Here's how the part is built. I have some questions about the finished solid (model axes, mm). Face numbers are marked on the shaded views. A direction names the side the tool comes from. Round coordinates to 2 decimals unless told otherwise and drop trailing zeros. Write each loop counter-clockwise with the first axis right and the second up, starting at its lowest first coordinate (ties: lowest second). Pieces come first, ordered by that corner, then holes. Notation, with made-up numbers: (41, 65.25) - (54, 65.25) arc R11 ccw to (54, 80.25) - close; hole circle Ø11 at (-15, -1.5). An arc over 180 degrees is marked (long way). One line per item, written item: value. Start each with the question number.
Item 1: Imagine slicing it at D-D, the plane z = 44. Count the separate pieces of the cut face and the enclosed holes in it, then the cut area to 3 significant figures.
Item 2: For the marked faces 1 and 2, which set-ups out of +Z, -Z, +X, -X, +Y, -Y let a thin tool reach every point of the face, with its end or its side?
Item 3: Thinking about a two-plate mould opening in X: for the marked faces 3, 4 and 5, which applies, released by +X, released by -X, zero draft, split by the parting line, or undercut?
Item 4: Imagine slicing it at A-A, the plane y = 0. Please give me the cut outline in (x, z).
Item 5: Imagine slicing it at C-C, the plane x = -42. Please give me the cut outline in (y, z).
Item 6: If I drill on line 1 (X direction, y = 40, z = 47.5); line 2 (X direction, y = 0.5, z = 47.75); line 3 (X direction, y = -34.5, z = 48.5), over which ranges is the centre line in solid material (lowest first)?
Item 7: For P1, Ø5, axis at x = -17.5, z = 49.5, coming from the +Y side; P2, Ø2, axis at y = -38.5, z = 46.5, coming from the +X side; P3, Ø2, axis at x = 43.5, z = 46, coming from the -Y side, each with a flat end and sliding along its axis, tell me the tip position at first contact or that it passes through.
```python
from build123d import *

# Parameters (mm, degrees)
CYLINDER469_R               = 1.5
CYLINDER469_DEPTH           = 100
CYLINDER472_R               = 1.5
CYLINDER472_DEPTH           = 100
CYLINDER472_ROLL_ANGLE      = -0.500355
CYLINDER472_PITCH_ANGLE     = 0.967193
CYLINDER472_PLACEMENT_ANGLE = 144.93646
CYLINDER481_R               = 1.5
CYLINDER481_DEPTH           = 100
CYLINDER476_R               = 1.5
CYLINDER476_DEPTH           = 100
CYLINDER476_PLACEMENT_ANGLE = 225
CYLINDER470_R               = 1.5
CYLINDER470_DEPTH           = 100
CYLINDER475_R               = 1.5
CYLINDER475_DEPTH           = 100
CYLINDER475_PLACEMENT_ANGLE = 45
CYLINDER479_R               = 1.5
CYLINDER479_DEPTH           = 100
CYLINDER479_ROLL_ANGLE      = 0.146073
CYLINDER479_PITCH_ANGLE     = 1.079101
CYLINDER479_PLACEMENT_ANGLE = -9.939308
CYLINDER471_R               = 1.5
CYLINDER471_DEPTH           = 100
CYLINDER471_PLACEMENT_ANGLE = 45
CYLINDER468_R               = 8
CYLINDER468_DEPTH           = 18
CYLINDER480_R               = 8
CYLINDER480_DEPTH           = 18
CYLINDER480_PLACEMENT_ANGLE = 225
CYLINDER483_R               = 8
CYLINDER483_DEPTH           = 18
CYLINDER482_R               = 8
CYLINDER482_DEPTH           = 18
CYLINDER482_ROLL_ANGLE      = -0.500355
CYLINDER482_PITCH_ANGLE     = 0.967193
CYLINDER482_PLACEMENT_ANGLE = 144.93646
CYLINDER474_R               = 8
CYLINDER474_DEPTH           = 18
CYLINDER478_R               = 8
CYLINDER478_DEPTH           = 18
CYLINDER478_PLACEMENT_ANGLE = 45
CYLINDER473_R               = 8
CYLINDER473_DEPTH           = 18
CYLINDER473_ROLL_ANGLE      = 0.146073
CYLINDER473_PITCH_ANGLE     = 1.079101
CYLINDER473_PLACEMENT_ANGLE = -9.939308
CYLINDER477_R               = 8
CYLINDER477_DEPTH           = 18
CYLINDER477_PLACEMENT_ANGLE = 45
TUBE025_R                   = 58
TUBE025_R_2                 = 30
TUBE025_DEPTH               = 10


with BuildPart() as obj1:
    # Cylinder469 → Cylinder469 (new body)
    with BuildSketch(Plane(origin=(38.80294, -16.072704, 0), x_dir=(0, 1, 0), z_dir=(0, 0, 1))):
        Circle(CYLINDER469_R)
    extrude(amount=CYLINDER469_DEPTH)


with BuildPart() as obj2:
    # Cylinder472 → Cylinder472 (new body)
    with BuildSketch(Plane.XY):
        Circle(CYLINDER472_R)
    extrude(amount=CYLINDER472_DEPTH)


with BuildPart() as obj2_1:
    # Cylinder472 roll: moved
    add(obj2.part.rotate(Axis((0, 0, 0), (1, 0, 0)), CYLINDER472_ROLL_ANGLE))


with BuildPart() as obj2_2:
    # Cylinder472 pitch: moved
    add(obj2_1.part.rotate(Axis((0, 0, 0), (0, 1, 0)), CYLINDER472_PITCH_ANGLE))


with BuildPart() as obj2_3:
    # Cylinder472 placement: moved
    add(obj2_2.part.moved(Location((35.440039, 22.530677, 0.610113))).rotate(Axis((35.440039, 22.530677, 0.610113), (0, 0, 1)), CYLINDER472_PLACEMENT_ANGLE))


with BuildPart() as obj3:
    # Cylinder481 → Cylinder481 (new body)
    with BuildSketch(Plane(origin=(16.072704, 38.80294, 0), x_dir=(-1, 0, 0), z_dir=(0, 0, 1))):
        Circle(CYLINDER481_R)
    extrude(amount=CYLINDER481_DEPTH)


with BuildPart() as obj4:
    # Cylinder476 → Cylinder476 (new body)
    with BuildSketch(Plane.XY):
        Circle(CYLINDER476_R)
    extrude(amount=CYLINDER476_DEPTH)


with BuildPart() as obj4_1:
    # Cylinder476 placement: moved
    add(obj4.part.moved(Location((-16.072704, 38.80294, 0))).rotate(Axis((-16.072704, 38.80294, 0), (0, 0, 1)), CYLINDER476_PLACEMENT_ANGLE))


with BuildPart() as obj5:
    # Cylinder470 → Cylinder470 (new body)
    with BuildSketch(Plane(origin=(-38.80294, 16.072704, 0), x_dir=(0, -1, 0), z_dir=(0, 0, 1))):
        Circle(CYLINDER470_R)
    extrude(amount=CYLINDER470_DEPTH)


with BuildPart() as obj6:
    # Cylinder475 → Cylinder475 (new body)
    with BuildSketch(Plane.XY):
        Circle(CYLINDER475_R)
    extrude(amount=CYLINDER475_DEPTH)


with BuildPart() as obj6_1:
    # Cylinder475 placement: moved
    add(obj6.part.moved(Location((-38.80294, -16.072704, 0))).rotate(Axis((-38.80294, -16.072704, 0), (0, 0, -1)), CYLINDER475_PLACEMENT_ANGLE))


with BuildPart() as obj7:
    # Cylinder479 → Cylinder479 (new body)
    with BuildSketch(Plane.XY):
        Circle(CYLINDER479_R)
    extrude(amount=CYLINDER479_DEPTH)


with BuildPart() as obj7_1:
    # Cylinder479 roll: moved
    add(obj7.part.rotate(Axis((0, 0, 0), (1, 0, 0)), CYLINDER479_ROLL_ANGLE))


with BuildPart() as obj7_2:
    # Cylinder479 pitch: moved
    add(obj7_1.part.rotate(Axis((0, 0, 0), (0, 1, 0)), CYLINDER479_PITCH_ANGLE))


with BuildPart() as obj7_3:
    # Cylinder479 placement: moved
    add(obj7_2.part.moved(Location((-22.528054, -35.446371, 0.203785))).rotate(Axis((-22.528054, -35.446371, 0.203785), (0, 0, 1)), CYLINDER479_PLACEMENT_ANGLE))


with BuildPart() as compound338:
    # Cylinder471 → Cylinder471 (new body)
    with BuildSketch(Plane.XY):
        Circle(CYLINDER471_R)
    extrude(amount=CYLINDER471_DEPTH)


with BuildPart() as compound338_1:
    # Cylinder471 placement: moved
    add(compound338.part.moved(Location((16.072704, -38.80294, 0))).rotate(Axis((16.072704, -38.80294, 0), (0, 0, 1)), CYLINDER471_PLACEMENT_ANGLE))

    # Compound338: union obj1, obj2, obj3, obj4, obj5, obj6, obj7
    add(obj1.part)
    add(obj2_3.part)
    add(obj3.part)
    add(obj4_1.part)
    add(obj5.part)
    add(obj6_1.part)
    add(obj7_3.part)


with BuildPart() as obj8:
    # Cylinder468 → Cylinder468 (new body)
    with BuildSketch(Plane(origin=(-38.798949, 16.072537, 43), x_dir=(0, -1, 0), z_dir=(0, 0, 1))):
        Circle(CYLINDER468_R)
    extrude(amount=CYLINDER468_DEPTH)


with BuildPart() as obj9:
    # Cylinder480 → Cylinder480 (new body)
    with BuildSketch(Plane.XY):
        Circle(CYLINDER480_R)
    extrude(amount=CYLINDER480_DEPTH)


with BuildPart() as obj9_1:
    # Cylinder480 placement: moved
    add(obj9.part.moved(Location((-16.07, 38.8, 43))).rotate(Axis((-16.07, 38.8, 43), (0, 0, 1)), CYLINDER480_PLACEMENT_ANGLE))


with BuildPart() as obj10:
    # Cylinder483 → Cylinder483 (new body)
    with BuildSketch(Plane(origin=(16.072537, 38.798949, 43), x_dir=(-1, 0, 0), z_dir=(0, 0, 1))):
        Circle(CYLINDER483_R)
    extrude(amount=CYLINDER483_DEPTH)


with BuildPart() as obj11:
    # Cylinder482 → Cylinder482 (new body)
    with BuildSketch(Plane.XY):
        Circle(CYLINDER482_R)
    extrude(amount=CYLINDER482_DEPTH)


with BuildPart() as obj11_1:
    # Cylinder482 roll: moved
    add(obj11.part.rotate(Axis((0, 0, 0), (1, 0, 0)), CYLINDER482_ROLL_ANGLE))


with BuildPart() as obj11_2:
    # Cylinder482 pitch: moved
    add(obj11_1.part.rotate(Axis((0, 0, 0), (0, 1, 0)), CYLINDER482_PITCH_ANGLE))


with BuildPart() as obj11_3:
    # Cylinder482 placement: moved
    add(obj11_2.part.moved(Location((34.627801, 22.637113, 43.602309))).rotate(Axis((34.627801, 22.637113, 43.602309), (0, 0, 1)), CYLINDER482_PLACEMENT_ANGLE))


with BuildPart() as obj12:
    # Cylinder474 → Cylinder474 (new body)
    with BuildSketch(Plane(origin=(38.798949, -16.072537, 43), x_dir=(0, 1, 0), z_dir=(0, 0, 1))):
        Circle(CYLINDER474_R)
    extrude(amount=CYLINDER474_DEPTH)


with BuildPart() as obj13:
    # Cylinder478 → Cylinder478 (new body)
    with BuildSketch(Plane.XY):
        Circle(CYLINDER478_R)
    extrude(amount=CYLINDER478_DEPTH)


with BuildPart() as obj13_1:
    # Cylinder478 placement: moved
    add(obj13.part.moved(Location((16.07, -38.8, 43))).rotate(Axis((16.07, -38.8, 43), (0, 0, 1)), CYLINDER478_PLACEMENT_ANGLE))


with BuildPart() as obj14:
    # Cylinder473 → Cylinder473 (new body)
    with BuildSketch(Plane.XY):
        Circle(CYLINDER473_R)
    extrude(amount=CYLINDER473_DEPTH)


with BuildPart() as obj14_1:
    # Cylinder473 roll: moved
    add(obj14.part.rotate(Axis((0, 0, 0), (1, 0, 0)), CYLINDER473_ROLL_ANGLE))


with BuildPart() as obj14_2:
    # Cylinder473 pitch: moved
    add(obj14_1.part.rotate(Axis((0, 0, 0), (0, 1, 0)), CYLINDER473_PITCH_ANGLE))


with BuildPart() as obj14_3:
    # Cylinder473 placement: moved
    add(obj14_2.part.moved(Location((-21.748471, -35.690226, 43.196026))).rotate(Axis((-21.748471, -35.690226, 43.196026), (0, 0, 1)), CYLINDER473_PLACEMENT_ANGLE))


with BuildPart() as compound336:
    # Cylinder477 → Cylinder477 (new body)
    with BuildSketch(Plane.XY):
        Circle(CYLINDER477_R)
    extrude(amount=CYLINDER477_DEPTH)


with BuildPart() as compound336_1:
    # Cylinder477 placement: moved
    add(compound336.part.moved(Location((-38.8, -16.07, 43))).rotate(Axis((-38.8, -16.07, 43), (0, 0, -1)), CYLINDER477_PLACEMENT_ANGLE))

    # Compound336: union obj8, obj9, obj10, obj11, obj12, obj13, obj14
    add(obj8.part)
    add(obj9_1.part)
    add(obj10.part)
    add(obj11_3.part)
    add(obj12.part)
    add(obj13_1.part)
    add(obj14_3.part)


with BuildPart() as compound336_2:
    # Compound336 placement: moved
    add(compound336_1.part.moved(Location((0, 0, 3))))


with BuildPart() as obj15:
    # Tube025 → Tube025 (new body)
    with BuildSketch(Plane.XY.offset(42)):
        Circle(TUBE025_R)
        Circle(TUBE025_R_2, mode=Mode.SUBTRACT)
    extrude(amount=TUBE025_DEPTH)

    # Cut173: cut Compound336
    add(compound336_2.part, mode=Mode.SUBTRACT)

    # Cut174: cut Compound338
    add(compound338_1.part, mode=Mode.SUBTRACT)


solid = obj15.part
```
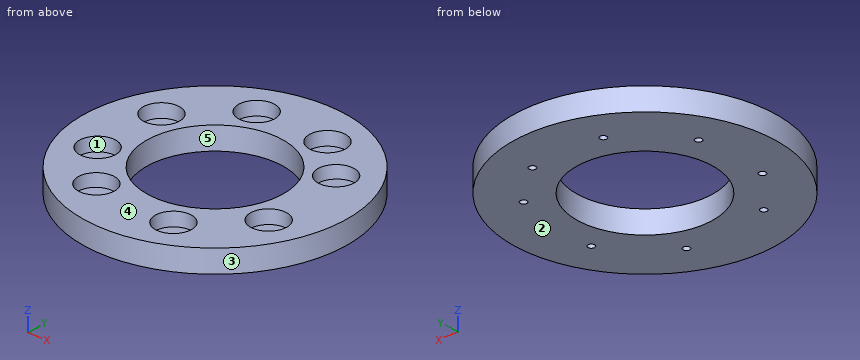
Values follow:
1. separate pieces: 1
1. enclosed holes: 9
1. area: 7,680 mm^2
2. face 1: +Z
2. face 2: -Z, +X, -X, +Y, -Y
3. face 3: split by the parting line
3. face 4: zero draft
3. face 5: undercut
4. outline: (-58, 42) - (-30, 42) - (-30, 52) - (-58, 52) - close; (30, 42) - (58, 42) - (58, 52) - (30, 52) - close
5. outline: (-40, 42) - (40, 42) - (40, 52) - (23.4, 52) - (23.4, 46) - (8.74, 46) - (8.74, 52) - (-8.74, 52) - (-8.74, 46) - (-23.4, 46) - (-23.4, 52) - (-40, 52) - close
6. line 1: x = -42 to -23.98, -8.16 to 8.16, 23.98 to 42
6. line 2: x = -58 to -30, 30 to 58
6. line 3: x = -46.62 to -29.62, -13.8 to 9.32, 22.82 to 46.62
7. P1: stops at y = 56.03
7. P2: stops at x = 44.25
7. P3: stops at y = -39.47
